The model under review builds one solid part; all positions refer to its coordinate system, in mm. Coordinates: 2 decimals unless noted, no trailing zeros. Write each loop counter-clockwise with the first axis right and the second up, starting at its lowest first coordinate (ties: lowest second). Pieces come first, ordered by that corner, then holes.
```python
from build123d import *

# Parameters (mm, degrees)
CROQUIS1_R                   = 3
SALIENTE_EXTRUIR1_DEPTH      = 390
CROQUIS2_R                   = 6
CROQUIS2_R_2                 = 3
SALIENTE_EXTRUIR5_DEPTH      = 9
SALIENTE_EXTRUIR5_DEPTH_BACK = 12
CROQUIS8_R                   = 3
SALIENTE_EXTRUIR6_DEPTH      = 9
CROQUIS9_R                   = 3
CORTAR_EXTRUIR1_DEPTH        = 10


with BuildPart() as part:
    # Croquis1 → Saliente-Extruir1 (new body)
    with BuildSketch(Plane(origin=(0, 0, 0), x_dir=(1, 0, 0), z_dir=(0, 1, 0))):
        Circle(CROQUIS1_R)
    extrude(amount=SALIENTE_EXTRUIR1_DEPTH)

    # Croquis2 → Saliente-Extruir5 (add, two sides)
    with BuildSketch(Plane(origin=(0, 390, 0), x_dir=(1, 0, 0), z_dir=(0, 1, 0))) as saliente_extruir5_sk:
        Circle(CROQUIS2_R)
        Circle(CROQUIS2_R_2, mode=Mode.SUBTRACT)
    extrude(amount=SALIENTE_EXTRUIR5_DEPTH)
    extrude(saliente_extruir5_sk.sketch, amount=-SALIENTE_EXTRUIR5_DEPTH_BACK)

    # Croquis8 → Saliente-Extruir6 (add)
    with BuildSketch(Plane(origin=(0, 390, 0), x_dir=(1, 0, 0), z_dir=(0, 1, 0))):
        Circle(CROQUIS8_R)
    extrude(amount=SALIENTE_EXTRUIR6_DEPTH)

    # Croquis9 → Cortar-Extruir1 (cut, symmetric)
    with BuildSketch(Plane.XY):
        with Locations((0, 393)):
            Circle(CROQUIS9_R)
    extrude(amount=CORTAR_EXTRUIR1_DEPTH, both=True, mode=Mode.SUBTRACT)


solid = part.part
```
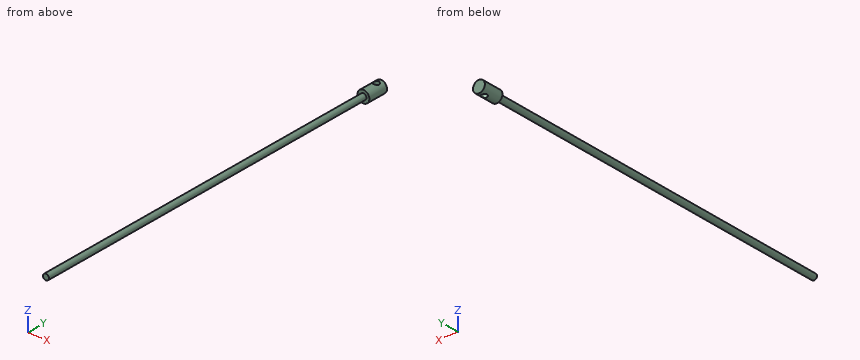
Item 1: Take a section at B-B, the plane z = 0. Write out the cut boundary in (x, y), plus the area to 3 significant figures.
Solved:
outline: (-6, 378) - (-3, 378) - (-3, 0) - (3, 0) - (3, 378) - (6, 378) - (6, 399) - (-6, 399) - close; hole circle Ø6 at (0, 393)
area: 2,490 mm2
Item 2: For pin 1 (5.5 mm diameter, centred on x = 0, y = 393, fed in from -Z); pin 2 (3 mm diameter, centred on x = 3.5, y = 182.5, fed in from +Z); pin 3 (5 mm diameter, centred on x = 4.5, y = 46.5, fed in from -Z); pin 4 (1.5 mm diameter, centred on x = 3.5, z = -2, fed in from -Y), all flat-tipped, find the tip position at first contact; note any pin that passes through.
Solved:
pin 1: passes through
pin 2: stops at z = 2.24
pin 3: stops at z = -2.24
pin 4: stops at y = 378
Item 3: Take a section at C-C, the plane y = 175.5. Write out the cut boundary in (x, z).
Solved:
outline: circle Ø6 at (0, 0)
Item 4: To check wall thickness, follow line 1 along Y through (x, z) = (0, 0); line 2 along Y through (x, z) = (4, -3.5); line 3 along X through (y, z) = (393, 0.75). State the ranges of each line that lie inside material, in increasing order.
Solved:
line 1: y = 0 to 390, 396 to 399
line 2: y = 378 to 399
line 3: x = -5.95 to -3, 3 to 5.95
Item 5: Take a section at A-A, the plane x = 0. Write out the cut boundary in (y, z), plus the area to 3 significant figures.
Solved:
outline: (0, -3) - (378, -3) - (378, -6) - (390, -6) - (390, 6) - (378, 6) - (378, 3) - (0, 3) - close; (396, -6) - (399, -6) - (399, 6) - (396, 6) - close
area: 2,450 mm2
